```python
from build123d import *

# Parameters (mm, degrees)
CROQUIS1_R              = 1.125
SALIENTE_EXTRUIR1_DEPTH = 2
CROQUIS3_W              = 7
CROQUIS3_H              = 2.5
SALIENTE_EXTRUIR2_DEPTH = 2


with BuildPart() as part:
    # Croquis1 → Saliente-Extruir1 (new body)
    with BuildSketch(Plane(origin=(0, 0, 0), x_dir=(1, 0, 0), z_dir=(0, 1, 0))):
        with BuildLine():
            Line((19.91, 0), (6.5, 0))
            Line((6.5, 0), (6.5, -3))
            Line((6.5, -3), (-6.5, -3))
            Line((-6.5, -3), (-6.5, 0))
            Line((-6.5, 0), (-19.91, 0))
            ThreePointArc((-19.91, 0), (-22.031320344, 0.878679656), (-22.91, 3))
            Line((-22.91, 3), (-22.91, 10))
            Line((-22.91, 10), (-21.51, 10))
            Line((-21.51, 10), (-21.51, 12))
            Line((-21.51, 12), (-18.51, 12))
            Line((-18.51, 12), (-18.51, 10))
            Line((-18.51, 10), (-14.51, 10))
            Line((-14.51, 10), (-14.51, 12))
            Line((-14.51, 12), (-11.51, 12))
            Line((-11.51, 12), (-11.51, 10))
            Line((-11.51, 10), (-9.01, 10))
            ThreePointArc((-9.01, 10), (-6.888679656, 9.121320344), (-6.01, 7))
            Line((-6.01, 7), (-6.01, 2))
            Line((-6.01, 2), (6.01, 2))
            Line((6.01, 2), (6.01, 7))
            ThreePointArc((6.01, 7), (6.888679656, 9.121320344), (9.01, 10))
            Line((9.01, 10), (11.51, 10))
            Line((11.51, 10), (11.51, 12))
            Line((11.51, 12), (14.51, 12))
            Line((14.51, 12), (14.51, 10))
            Line((14.51, 10), (18.51, 10))
            Line((18.51, 10), (18.51, 12))
            Line((18.51, 12), (21.51, 12))
            Line((21.51, 12), (21.51, 10))
            Line((21.51, 10), (22.91, 10))
            Line((22.91, 10), (22.91, 3))
            ThreePointArc((22.91, 3), (22.031320344, 0.878679656), (19.91, 0))
        make_face()
        with Locations(Location((-16.51, 3.5, 0), (0, 0, 270))):
            Circle(CROQUIS1_R, mode=Mode.SUBTRACT)
        with Locations(Location((16.51, 3.5, 0), (0, 0, 90))):
            Circle(CROQUIS1_R, mode=Mode.SUBTRACT)
    extrude(amount=SALIENTE_EXTRUIR1_DEPTH)

    # Croquis3 → Saliente-Extruir2 (add)
    with BuildSketch(Plane.XZ):
        with Locations((-16.51, -6.75)):
            Rectangle(CROQUIS3_W, CROQUIS3_H)
        with Locations((16.51, -6.75)):
            Rectangle(CROQUIS3_W, CROQUIS3_H)
    extrude(amount=SALIENTE_EXTRUIR2_DEPTH)


solid = part.part
```
Here's how the part is built. I have some questions about the finished solid (model axes, mm). A direction names the side the tool comes from. Round coordinates to 2 decimals unless told otherwise and drop trailing zeros. Order: outer loops, then holes, each group sorted by start corner. A loop starts at its lowest first (then second) coordinate and runs counter-clockwise, first axis right, second up. Notation, with made-up numbers: (89.25, 50.5) -> (141.25, 50.5) arc R13 cw to (141.25, 58.5) -> close; hole circle Ø1 at (56, 60). An arc over 180 degrees is marked (long way). Use a Markdown table: item, result. Add a question column.
(1) Suppose I cut it at B-B, the plane x = 16.51. Please give me the cut outline in (y, z) (3 decimals).
(2) I need wall thicknesses on line 1 along X through (y, z) = (0.95, -3.5) (3 decimals); line 2 along Z through (x, y) = (16.51, 1.5) (3 decimals); line 3 along X through (y, z) = (1.6, -6.5). Which ranges of each line are inside material? Lowest first, please.
(3) For pin 1 Ø0.6 at (x, y) = (3, 1) entering from -Z; pin 2 Ø0.6 at (y, z) = (-1, -6.5) entering from -X; pin 3 Ø0.6 at (y, z) = (1, 2) entering from +X, each with a flat end and sliding along its axis, tell me the tip position at first contact or that it passes through.
(4) Suppose I cut it at C-C, the plane x = -19. Please give me the cut outline in (y, z).
(5) For faces 1 (the face through (21.51, 1, -11)), 2 (the face through (-22, 1, -10)), 3 (the face through (-17, -1, -5.5)), 4 (the face through (-6.91, 0.99, -9.14)), 5 (the face through (13, 1, 0)), which set-ups out of +Z, -Z, +X, -X, +Y, -Y let a thin tool reach every point of the face, with its end or its side?
(6) Suppose I cut it at A-A, the plane z = -11. Please give me the cut outline in (x, y), and give its area (3 significant figures).
(7) Suppose I cut it at D-D, the plane z = -3.5. Please give me the cut outline in (x, y) (3 decimals).
(8) If we mould it in two halves opening along Z, with no side actions, what happens to faces 6 (the face through (14.51, 1, -11)), 7 (the face through (15.395, 0.986, -3.354)), 8 (the face through (-17, -1, -8))? For each: released by +Z, released by -Z, zero draft, split by the parting line, or undercut.
Verdict:
| question | item | result |
|---|---|---|
| 1 | outline | (-2, -8) -> (0, -8) -> (0, -10) -> (2, -10) -> (2, -4.625) -> (0, -4.625) -> (0, -5.5) -> (-2, -5.5) -> close; (0, -2.375) -> (2, -2.375) -> (2, 0) -> (0, 0) -> close |
| 2 | line 1 | -22.91 to -17.635, -15.385 to -6.01, 6.01 to 15.385, 17.635 to 22.91 |
| 2 | line 2 | -10 to -4.625, -2.375 to 0 |
| 2 | line 3 | -22.91 to -6.01, 6.01 to 22.91 |
| 3 | pin 1 | z = -2 |
| 3 | pin 2 | x = -20.01 |
| 3 | pin 3 | x = 6.5 |
| 4 | outline | (-2, -8) -> (0, -8) -> (0, -12) -> (2, -12) -> (2, 0) -> (0, 0) -> (0, -5.5) -> (-2, -5.5) -> close |
| 5 | face 1 | -Z, +X, +Y, -Y |
| 5 | face 2 | -Z, -X, +Y, -Y |
| 5 | face 3 | +Z, +X, -X, -Y |
| 5 | face 4 | -Z, +Y, -Y |
| 5 | face 5 | +Z, +X, +Y, -Y |
| 6 | outline | (-21.51, 0) -> (-18.51, 0) -> (-18.51, 2) -> (-21.51, 2) -> close; (-14.51, 0) -> (-11.51, 0) -> (-11.51, 2) -> (-14.51, 2) -> close; (11.51, 0) -> (14.51, 0) -> (14.51, 2) -> (11.51, 2) -> close; (18.51, 0) -> (21.51, 0) -> (21.51, 2) -> (18.51, 2) -> close |
| 6 | area | 24.0 mm2 |
| 7 | outline | (-22.91, 0) -> (-17.635, 0) -> (-17.635, 2) -> (-22.91, 2) -> close; (-15.385, 0) -> (-6.01, 0) -> (-6.01, 2) -> (-15.385, 2) -> close; (6.01, 0) -> (15.385, 0) -> (15.385, 2) -> (6.01, 2) -> close; (17.635, 0) -> (22.91, 0) -> (22.91, 2) -> (17.635, 2) -> close |
| 8 | face 6 | zero draft |
| 8 | face 7 | undercut |
| 8 | face 8 | released by -Z |
